Source: CAD feature listing. Evaluate the final solid. Frame: model axes, mm. A direction names the side the tool comes from. Round coordinates to 2 decimals unless told otherwise and drop trailing zeros. Loops run counter-clockwise (first coordinate to the right, second up) from the corner with the lowest first, then second, coordinate; pieces in that order, holes last. Notation, with made-up numbers: (23, 49) -> (39, 49) arc R28 ccw to (39, 82) -> close; hole circle Ø3 at (-29.75, 72). An arc over 180 degrees is marked (long way). Write item = value, one per line.
from build123d import *

# Parameters (mm, degrees)
F0_R     = 36.593619
F1_DEPTH = 25.4
F3_R     = 5.460111
F4_DEPTH = 76.708
F5_W     = 35.531597
F5_H     = 58.026424
F6_DEPTH = 22.098


with BuildPart() as f1:
    # F0 (on Top) → F1 (new body)
    with BuildSketch(Plane.XY):
        Circle(F0_R)
    extrude(amount=F1_DEPTH)

    # F3 (on offset) → F4 (cut)
    with BuildSketch(Plane.XZ.offset(-37.084)):
        with Locations((0, 13.036774)):
            Circle(F3_R)
    extrude(amount=F4_DEPTH, mode=Mode.SUBTRACT)

    # F5 (on Top) → F6 (cut)
    with BuildSketch(Plane.XY):
        with Locations((0.766869, -0.383434)):
            Rectangle(F5_W, F5_H)
    extrude(amount=F6_DEPTH, mode=Mode.SUBTRACT)


solid = f1.part
1. Line query: probe 1 along Z at (x, y) = (0, -32); probe 2 along Y at (x, z) = (-0.5, 1.25); probe 3 along X at (y, z) = (-3, 12.25). Output: solid intervals per line, ascending. Write a range as from..to.
Evaluation:
probe_1 = 0..7.58, 18.5..25.4
probe_2 = -36.59..-29.4, 28.63..36.59
probe_3 = -36.47..-17, 18.53..36.47
2. Section query B-B (y = 0). Return the cut outline in (x, z), then the cut area to 3 significant figures.
Evaluation:
outline = (-36.59, 0) -> (-17, 0) -> (-17, 22.1) -> (18.53, 22.1) -> (18.53, 0) -> (36.59, 0) -> (36.59, 25.4) -> (-36.59, 25.4) -> close
area = 1,070 mm²
3. Set-up query: faces 4 (the face through (-1, 1, 25.4)), 5 (the face through (1, 0, 22.098)). Return all of +Z, -Z, +X, -X, +Y, -Y with unobstructed straight access to the full face (end or side cutting, diameter ignored); none if empty.
Evaluation:
face_4 = +Z, +X, -X, +Y, -Y
face_5 = -Z
4. Mould query, pull axis X, two halves, no side actions, for faces 1 (the face through (-7.933, -35.723, 12.522)), 2 (the face through (4, -29.397, 8)), 3 (the face through (24, 1, 0)). Classes: released by +X, released by -X, zero draft, split by the parting line, or undercut.
Evaluation:
face_1 = split by the parting line
face_2 = undercut
face_3 = zero draft
5. Section query C-C (z = 4). Return the cut outline in (x, y), then the cut area to 3 significant figures.
Evaluation:
outline = circle Ø73.19 at (0, 0); hole (-17, -29.4) -> (18.53, -29.4) -> (18.53, 28.63) -> (-17, 28.63) -> close
area = 2,150 mm²
6. Contact query for flat-ended pins moving along their axis: pin 1 Ø5 at (x, z) = (17.5, 15.5) entering from +Y; pin 2 Ø4 at (x, y) = (9, -11.5) entering from -Z; pin 3 Ø4 at (x, z) = (-17.5, 15.5) entering from -Y. Output: stop coordinate, or through.
Evaluation:
pin_1 = 33.38
pin_2 = 22.1
pin_3 = -33.15
7. Section query D-D (z = 17.5). Return the cut outline in (x, y).
Evaluation:
outline = (-17, -29.4) -> (-17, 28.63) -> (-3.15, 28.63) -> (-3.15, 36.46) arc R36.59 ccw to (-3.15, -36.46) -> (-3.15, -29.4) -> close; (3.15, -36.46) arc R36.59 ccw to (3.15, 36.46) -> (3.15, 28.63) -> (18.53, 28.63) -> (18.53, -29.4) -> (3.15, -29.4) -> close
8. Section query A-A (x = 0). Return the cut outline in (y, z), then the cut area to 3 significant figures.
Evaluation:
outline = (-36.59, 0) -> (-29.4, 0) -> (-29.4, 7.58) -> (-36.59, 7.58) -> close; (-36.59, 18.5) -> (-29.4, 18.5) -> (-29.4, 22.1) -> (28.63, 22.1) -> (28.63, 18.5) -> (36.59, 18.5) -> (36.59, 25.4) -> (-36.59, 25.4) -> close; (28.63, 0) -> (36.59, 0) -> (36.59, 7.58) -> (28.63, 7.58) -> close
area = 411 mm²
